Geometry check sheet. Reference: the model listing, model coordinates, mm. A direction names the side the tool comes from. Coordinates: 2 decimals unless noted, no trailing zeros. Write each loop counter-clockwise with the first axis right and the second up, starting at its lowest first coordinate (ties: lowest second). Pieces come first, ordered by that corner, then holes. Notation, with made-up numbers: (-1.5, 61.25) -> (2.5, 61.25) arc R16 ccw to (2.5, 72.25) -> close; hole circle Ø2 at (22, 59.25). An arc over 180 degrees is marked (long way). Put each result on its own line as item: value. Start each with the question number.
from build123d import *

# Parameters (mm, degrees)
SKETCH_1_R      = 6.1
SKETCH_1_R_2    = 10.6
EXTRUDE_1_DEPTH = 8


with BuildPart() as part:
    # 草圖1 → 填料-伸長1 (new body)
    with BuildSketch(Plane.XY):
        with BuildLine():
            Line((-42.684704159, 14.986968014), (26.753169389, -13.357021069))
            Line((26.753169389, -13.357021069), (17.305173028, -36.502978918))
            Line((17.305173028, -36.502978918), (-24.357551101, -19.496585468))
            Line((-24.357551101, -19.496585468), (-40.005369853, -57.831036438))
            ThreePointArc((-40.005369853, -57.831036438), (-58.274878096, -62.897218292), (-67.780519272, -46.493440805))
            Line((-67.780519272, -46.493440805), (-42.684704159, 14.986968014))
        make_face()
        with Locations((-33.52112763, -2.254808727)):
            Circle(SKETCH_1_R, mode=Mode.SUBTRACT)
        with Locations((-52.417120352, -48.546724426)):
            Circle(SKETCH_1_R_2, mode=Mode.SUBTRACT)
        Polygon((1.043977728, -21.494495956), (4.634216345, -12.699031974), (14.046430901, -11.41053783), (19.868406839, -18.91750767), (16.278168222, -27.712971653), (6.865953666, -29.001465796), align=None, mode=Mode.SUBTRACT)
    extrude(amount=-EXTRUDE_1_DEPTH)


solid = part.part
Item 1: Section check C-C, the plane z = -1.75. Enter the section's corners in (x, y), and give its area (3 significant figures).
Item 2: Mould release check, pull along Y, two halves, no side actions. Record for faces 1 (the flat face through (9.274, -12.064, -3.944)), 2 (the flat face through (-27, -21, 0)), 3 (the flat face through (-55.408, -16.184, -3.944)), 4 (the flat face through (11.638, -28.348, -3.944)): released by +Y, released by -Y, zero draft, split by the parting line, or undercut.
Item 3: Section check B-B, the plane y = -30. Enter the section's corners in (x, z), and give its area (3 significant figures).
Item 4: Access from +Z, -Z, +X, -X, +Y, -Y to the whole of each face (thin tool, end or side, straight path). Record for faces 5 (the flat face through (3.996, -25.301, -3.944)), 6 (the flat face through (-27, -21, -8)), 7 (the flat face through (-32.072, -38.395, -3.944)).
Item 5: Scan lines: line 1 along Y through (x, z) = (-39, -7); line 2 along X through (y, z) = (-42.5, -3); line 3 along X through (y, z) = (-40, -4). Record each from-to range of solid material in increasing order. Write a range as [from, to].
Item 6: Section check A-A, the plane x = 2.5. Enter the section's corners in (y, z), and give its area (3 significant figures).
Item 7: Go/stop test with flat-tipped pins: P1, Ø1.5, axis at x = -29, z = -5.5, coming from the -Y side; P2, Ø1.5, axis at y = -22.5, z = -6.5, coming from the +X side; P3, Ø1.5, axis at x = 10, z = -4.5, coming from the +Y side. Record where each tip stops, or that it passes through.
From the geometry:
1. outline: (-67.78, -46.49) arc R15.5 ccw to (-40.01, -57.83) -> (-24.36, -19.5) -> (17.31, -36.5) -> (26.75, -13.36) -> (-42.68, 14.99) -> close; hole circle Ø21.2 at (-52.42, -48.55); hole circle Ø12.2 at (-33.52, -2.25); hole (1.04, -21.49) -> (6.87, -29) -> (16.28, -27.71) -> (19.87, -18.92) -> (14.05, -11.41) -> (4.63, -12.7) -> close
1. area: 2,670 mm²
2. face 1: undercut
2. face 2: zero draft
2. face 3: released by +Y
2. face 4: undercut
3. outline: (-61.05, -8) -> (-28.64, -8) -> (-28.64, 0) -> (-61.05, 0) -> close; (1.37, -8) -> (19.96, -8) -> (19.96, 0) -> (1.37, 0) -> close
3. area: 408 mm²
4. face 5: +Z, -Z
4. face 6: -Z, +X, -X, +Y, -Y
4. face 7: +Z, -Z, -Y
5. line 1: [-55.37, -4.94], [0.43, 13.48]
5. line 2: [-66.15, -61.12], [-43.71, -33.75]
5. line 3: [-65.13, -58.69], [-46.15, -32.73]
6. outline: (-30.46, -8) -> (-23.37, -8) -> (-23.37, 0) -> (-30.46, 0) -> close; (-17.93, -8) -> (-3.46, -8) -> (-3.46, 0) -> (-17.93, 0) -> close
6. area: 172 mm²
7. P1: y = -32.71
7. P2: x = 23.33
7. P3: y = -6.21
